The listing builds one solid part. Answer for the finished solid, in the listing's coordinates (mm). Face numbers are marked on the shaded views. A direction names the side the tool comes from. Coordinates: 2 decimals unless noted, no trailing zeros. Loops run counter-clockwise (first coordinate to the right, second up) from the corner with the lowest first, then second, coordinate; pieces in that order, holes last. Notation, with made-up numbers: (74, 79) - (115, 79) arc R27 ccw to (115, 114) - close; hole circle Ø2 at (-31.75, 61). An arc over 180 degrees is marked (long way). Put each result on its own line as item: value.
Autodesk Inventor part; units mm, degrees
ref_plane "Work Plane1" through (29, 0, 0) normal (0, -1, 0) x (1, 0, 0)
ref_plane "YZ Plane" through (0, 0, 0) normal (1, 0, 0) x (0, 1, 0)
ref_plane "XZ Plane" through (0, 0, 0) normal (0, 1, 0) x (-1, 0, 0)
sketch "Sketch1" plane through (0, 0, 0) normal (0, 0, 1) x (1, 0, 0)
  line L0 (0.1667, 0) -> (20, 0)
  line L1 (20, 0) -> (20, 1.5)
  line L2 (20, 1.5) -> (8, 1.5)
  line L3 (8, 1.5) -> (7.6932, 1.5)
  line L4 (7.6932, 1.5) -> (0, 1.5)
  line L5 (0, 1.5) -> (0, 2.75)
  line L6 (0, 2.75) -> (-2, 2.75)
  line L7 (-2, 2.75) -> (-2, 1.1547)
  line L8 (-2, 1.1547) -> (-0.5, 1.1547)
  line L9 (-0.5, 1.1547) -> (0.1667, 0)
  line L10 (-6.4, 0) -> (24.4, 0)
  line L11 (0, -0.55) -> (0, 3.3)
  line L12 (8, 1.5) -> (0, 1.5) construction
  dimension "d1" = 12
  dimension "d2" = 0.3068
  dimension "d3" = 2
  dimension "d4" = 1.5
  dimension "d5" = 60
  dimension "d6" = 3
  dimension "d7" = 3
  dimension "d8" = 2.3094
  dimension "d9" = 5.5
  dimension "d26" = 20
revolve "Body" add sketch "Sketch1" angle 360 about axis through (0.1667, 0, 0) along (1, 0, 0) contours L9 L11 L4 L3 L2 L1 L0 | L9 L8 L7 L6 L5 L11
sketch "Sketch2" plane through (-2, 0, 0) normal (-1, 0, 0) x (0, 0, 1)
  circle A0 centre (0, 0) radius 1.1547
  line L0 (0, -3.85) -> (0, 3.85)
  line L1 (-3.85, 0) -> (3.85, 0)
  line L2 (1.1547, 0) -> (0.5774, -1)
  line L3 (0.5774, -1) -> (-0.5774, -1)
  line L4 (-0.5774, -1) -> (-1.1547, 0)
  line L5 (-1.1547, 0) -> (-0.5774, 1)
  line L6 (-0.5774, 1) -> (0.5774, 1)
  line L7 (0.5774, 1) -> (1.1547, 0)
  point P0 (0, 0)
extrude "Slot" add sketch "Sketch2" against normal up to next contours L7 A0 | A0 L2 | L6 L0 A0 | A0 L0 L3 | L0 L6 A0 | A0 L3 L0 | L4 A0 | A0 L5
fillet "Fillet1" radius 0.3 1 edges at (-2, -2.75, 0)
thread "Thread"
chamfer "Chamfer1" distance 0.3067 distance2 0.3067 1 edges at (20, -1.5, 0) measured on face at (20, -0.7567, -0.3972)
ref_plane "Work Plane1" through (29, 0, 0) normal (0, -1, 0) x (1, 0, 0)
fillet "Fillet2" radius 0.1 1 edges at (0, -1.5, 0)
equation "\"d1\" = GEL"
equation "\"d3\" = KOH"
equation "\"d4\" = INTI"
equation "\"d6\" = GD"
equation "\"d7\" = BDM"
equation "\"d8\" = 1.1547 * SW"
equation "\"d9\" = KOD"
equation "\"d26\" = NLG"
equation "\"d30\" = R"
equation "\"d17\" = RR"
equation "\"d13\" = GEL"
equation "\"d15\" = -0.5 * SPD + 0.5 * GD"
equation "\"d16\" = GUL"
equation "\"GD\" = NND"
equation "\"NLG\" = 20"
equation "\"GEL\" = 12"
equation "\"KOD\" = 5.5"
equation "\"KOH\" = 2"
equation "\"INTI\" = 1.5"
equation "\"GAL\" = 0.61345 * PTC"
equation "\"GUL\" = 0.61345 * PTC"
equation "\"BDM\" = NND"
equation "\"SW\" = 2"
equation "\"RR\" = 0.3"
equation "\"SPD\" = NND - 1.2269 * PTC"
equation "\"R\" = 0.1"
equation "\"TOA\" = 30deg"
equation "\"GD1\" = THREADDIA - 1.2269 * PTC"
equation "\"THREADDIA\" = 3"
equation "\"FAWI\" = 45deg"
equation "\"ANG\" = 120deg"
equation "\"PTC\" = 0.5"
equation "\"NND\" = 3"
equation "\"E0\" = 1.155 * SW"
properties part number "DIN 7984 - M3 x 20" material "Steel, Mild"
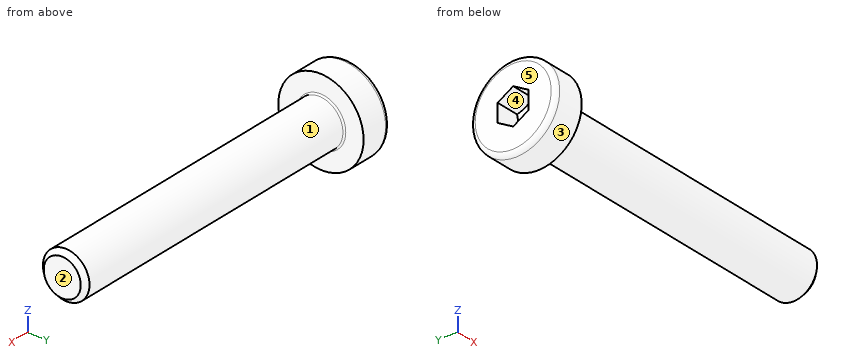
1) The part is cut by section A-A (x = 5.5). Give the vertices of the cut face in (y, z).
Found:
outline: circle Ø3 at (0, 0)
2) Each of these flat-tipped pins is pushed along its axis until it touches: pin 1 (1 mm diameter, centred on y = -0.5, z = -1.5, fed in from +X); pin 2 (2 mm diameter, centred on x = 9.5, y = 2, fed in from +Z); pin 3 (1 mm diameter, centred on x = 12.5, y = 1, fed in from +Z). Where does it stop, or does it pass through?
Found:
pin 1: stops at x = 20
pin 2: stops at z = 1.12
pin 3: stops at z = 1.41
3) For a pull along Z with two mould halves and no side action, classify the marked faces 3, 4 and 5 as pulls with the +Z half, pulls with the -Z half, needs draft (parallel to the pull), parting line crosses it, or undercut.
Found:
face 3: parting line crosses it
face 4: undercut
face 5: needs draft
4) Straight lines are drawn through the part: L1, parallel to X at y = -0.7, z = 1.5; L2, parallel to Z at x = 15.5, y = 0.1; L3, parallel to Y at x = 10.5, z = 1.05. For each, find the intervals that lie inside material, in ascending order. Write a range as [from, to].
Found:
L1: x = [-2, 0]
L2: z = [-1.5, 1.5]
L3: y = [-1.07, 1.07]
5) For the marked faces 1 and 2, determine the directions among +Z, -Z, +X, -X, +Y, -Y from which every point of the face is accessible in a straight line to the end or side of a thin tool.
Found:
face 1: +X
face 2: +Z, -Z, +X, +Y, -Y
